Can you work these out from the model? Positions are in its coordinate system, mm. Round coordinates to 2 decimals unless told otherwise and drop trailing zeros. Loops run counter-clockwise (first coordinate to the right, second up) from the corner with the lowest first, then second, coordinate; pieces in that order, holes last. Notation, with made-up numbers: (34, 37) -> (81, 37) arc R32 ccw to (81, 71) -> close; hole circle Ø8 at (-35, 33). An arc over 180 degrees is marked (long way). Answer as a JSON object with one key per item and string values.
```python
from build123d import *

# Parameters (mm, degrees)
CUT_EXTRUDE1_DEPTH      = 29.752043406
CUT_EXTRUDE1_DEPTH_BACK = 29.752043406
SKETCH3_W               = 19.816571208
SKETCH3_H               = 17.600838627
CUT_EXTRUDE2_DEPTH      = 29.448858181
SKETCH6_R               = 7.6
CUT_EXTRUDE3_DEPTH      = 29.734648075


with BuildPart() as part:
    # Sketch1 → Revolve1 (revolve)
    with BuildSketch(Plane.XY):
        with BuildLine():
            Line((0, 16.6), (0, -16.6))
            ThreePointArc((0, -16.6), (-16.6, 0), (0, 16.6))
        make_face()
    revolve(axis=Axis((0, 16.6, 0), (0, -1, 0)))

    # Sketch2 → Cut-Extrude1 (cut, two sides: drawn at the far end of the back side and taken through both)
    with BuildSketch(Plane(origin=(0, 0, 0), x_dir=(1, 0, 0), z_dir=(0, 1, 0)).offset(-CUT_EXTRUDE1_DEPTH_BACK)):
        with BuildLine():
            Line((-0.5, 16.592468171), (-0.5, 0.5))
            Line((-0.5, 0.5), (-16.592468171, 0.5))
            ThreePointArc((-16.592468171, 0.5), (11.737972568, -11.737972568), (-0.5, 16.592468171))
        make_face()
    extrude(amount=CUT_EXTRUDE1_DEPTH + CUT_EXTRUDE1_DEPTH_BACK, mode=Mode.SUBTRACT)

    # Sketch3 → Cut-Extrude2 (cut, through all)
    with BuildSketch(Plane(origin=(-0.5, 0, 0), x_dir=(0, 0, -1), z_dir=(1, 0, 0))):
        with Locations((9.908285604, -8.800419314)):
            Rectangle(SKETCH3_W, SKETCH3_H)
    extrude(amount=-CUT_EXTRUDE2_DEPTH, mode=Mode.SUBTRACT)

    # Sketch6 → Cut-Extrude3 (cut, through all)
    with BuildSketch(Plane.XZ):
        Circle(SKETCH6_R)
    extrude(amount=-CUT_EXTRUDE3_DEPTH, mode=Mode.SUBTRACT)


solid = part.part
```
Q1. I want a section at C-C, the plane x = -13.25. Write out the boundary of the cut face in (y, z).
Determined:
{"outline": "(0, -10) arc R10 ccw to (9.99, -0.5) -> (0, -0.5) -> close"}
Q2. If I drill on L1, parallel to Z at x = -4.25, y = 12.5; L2, parallel to X at y = 3, z = -2; L3, parallel to Z at x = -2, y = 9.75, over which ranges is the centre line in solid material (lowest first)? Write a range as [from, to].
Determined:
{"L1": "[-10.06, -6.3]", "L2": "[-16.2, -7.33]", "L3": "[-13.29, -7.33]"}
Q3. I want a section at B-B, the plane y = 12. Write out the boundary of the cut face in (x, z).
Determined:
{"outline": "(-11.46, -0.5) arc R11.47 ccw to (-0.5, -11.46) -> (-0.5, -7.58) arc R7.6 cw to (-7.58, -0.5) -> close"}
Q4. I want a section at A-A, the plane z = -3. Write out the boundary of the cut face in (x, y), then the cut area to 3 significant figures.
Determined:
{"outline": "(-16.33, 0) -> (-6.98, 0) -> (-6.98, 14.76) arc R16.33 ccw to start", "area": "98.9 mm²"}
Q5. I want a section at D-D, the plane y = 9.25. Write out the boundary of the cut face in (x, z).
Determined:
{"outline": "(-13.77, -0.5) arc R13.78 ccw to (-0.5, -13.77) -> (-0.5, -7.58) arc R7.6 cw to (-7.58, -0.5) -> close"}
Q6. I'm going to push flat-ended pins straight in: pin 1 (5 mm diameter, centred on x = -4, y = 9.5, fed in from +Z); pin 2 (2 mm diameter, centred on y = 5.5, z = -2.5, fed in from +X); pin 3 (5 mm diameter, centred on x = -8.5, y = 12.5, fed in from -Z). Where does each tip first touch, or does it pass through?
Determined:
{"pin 1": "z = -3.94", "pin 2": "x = -6.75", "pin 3": "z = -10.79"}
